Geometry check sheet. Reference: the model listing, model coordinates, mm. Give positions to 0.01 mm unless a question says otherwise; leave off trailing zeros. Write each loop counter-clockwise with the first axis right and the second up, starting at its lowest first coordinate (ties: lowest second). Pieces come first, ordered by that corner, then holes. Notation, with made-up numbers: M 32,8.5 L 65,8.5 A38 ccw 65,47.5 Z; hole C 46.25,75.5 d5. An arc over 180 degrees is marked long. One line per item, written item: value. Start each with the question number.
1. Scan lines: line 1 (Y direction, x = 32.5, z = 5); line 2 (X direction, y = -34, z = 3.75); line 3 (X direction, y = 53.5, z = 1). Record each from-to range of solid material in increasing order.
2. Gauge pin test, flat ends, axial feed: pin 1 (1.8 mm diameter, centred on x = -11, y = -54, fed in from -Z); pin 2 (2 mm diameter, centred on y = 58, z = 3.5, fed in from -X). Record the tip position at first contact, or that the pin passes through.
3. Cross-section at D-D on y = -29. Record the cut outline in (x, z).
4. Cross-section at A-A on y = 0. Record the cut outline in (x, z), then the cut area to 3 significant figures.
5. Cross-section at C-C on z = 4. Count the separate pieces of the cut face and the enclosed holes in it, then the cut area to 3 significant figures.
from build123d import *

# Parameters (mm, degrees)
SKETCH1_R           = 76.2
SKETCH1_R_2         = 2.25
SKETCH1_R_3         = 1.5
SKETCH1_R_4         = 1
SKETCH1_W           = 25.4
SKETCH1_H           = 25.4
BOSS_EXTRUDE2_DEPTH = 6.35
FILLET3_R           = 1
FILLET4_R           = 1
FILLET5_R           = 1
FILLET6_R           = 1


with BuildPart() as part:
    # Sketch1 → Boss-Extrude2 (new body)
    with BuildSketch(Plane.XY):
        Circle(SKETCH1_R)
        with Locations((-32.5, 29)):
            Circle(SKETCH1_R_2, mode=Mode.SUBTRACT)
        with Locations((-32.5, -29)):
            Circle(SKETCH1_R_2, mode=Mode.SUBTRACT)
        with Locations((32.5, -29)):
            Circle(SKETCH1_R_2, mode=Mode.SUBTRACT)
        with Locations((32.5, 29)):
            Circle(SKETCH1_R_2, mode=Mode.SUBTRACT)
        with Locations((43.5, 35)):
            Circle(SKETCH1_R_3, mode=Mode.SUBTRACT)
        with Locations((-43.5, 35)):
            Circle(SKETCH1_R_3, mode=Mode.SUBTRACT)
        with Locations((43.5, -35)):
            Circle(SKETCH1_R_3, mode=Mode.SUBTRACT)
        with Locations((-43.5, -35)):
            Circle(SKETCH1_R_3, mode=Mode.SUBTRACT)
        with Locations((-11, 54)):
            Circle(SKETCH1_R_4, mode=Mode.SUBTRACT)
        with Locations((11, 54)):
            Circle(SKETCH1_R_4, mode=Mode.SUBTRACT)
        with Locations((11, 62)):
            Circle(SKETCH1_R_4, mode=Mode.SUBTRACT)
        with Locations((-11, 62)):
            Circle(SKETCH1_R_4, mode=Mode.SUBTRACT)
        with Locations((-11, -62)):
            Circle(SKETCH1_R_4, mode=Mode.SUBTRACT)
        with Locations((-11, -54)):
            Circle(SKETCH1_R_4, mode=Mode.SUBTRACT)
        with Locations((11, -62)):
            Circle(SKETCH1_R_4, mode=Mode.SUBTRACT)
        with Locations((11, -54)):
            Circle(SKETCH1_R_4, mode=Mode.SUBTRACT)
        Rectangle(SKETCH1_W, SKETCH1_H, mode=Mode.SUBTRACT)
    extrude(amount=BOSS_EXTRUDE2_DEPTH)

    # Fillet3
    fillet3_edges = [part.edges().sort_by_distance(p)[0] for p in [
        (-12.7, -12.7, 3.175),
    ]]
    fillet(fillet3_edges, radius=FILLET3_R)

    # Fillet4
    fillet4_edges = [part.edges().sort_by_distance(p)[0] for p in [
        (12.7, 12.7, 3.175),
    ]]
    fillet(fillet4_edges, radius=FILLET4_R)

    # Fillet5
    fillet5_edges = [part.edges().sort_by_distance(p)[0] for p in [
        (-12.7, 12.7, 3.175),
    ]]
    fillet(fillet5_edges, radius=FILLET5_R)

    # Fillet6
    fillet6_edges = [part.edges().sort_by_distance(p)[0] for p in [
        (12.7, -12.7, 3.175),
    ]]
    fillet(fillet6_edges, radius=FILLET6_R)


solid = part.part
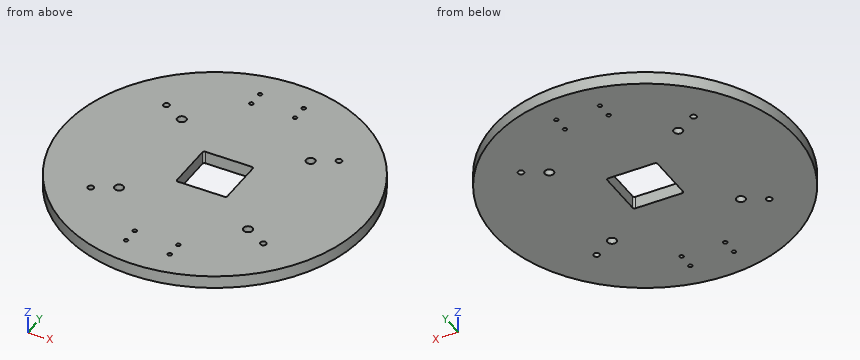
Report:
1. line 1: y = -68.92 to -31.25, -26.75 to 26.75, 31.25 to 68.92
1. line 2: x = -68.19 to -44.62, -42.38 to 42.38, 44.62 to 68.19
1. line 3: x = -54.26 to -11.87, -10.13 to 10.13, 11.87 to 54.26
2. pin 1: passes through
2. pin 2: stops at x = -50.57
3. outline: M -70.47,0 L -34.75,0 L -34.75,6.35 L -70.47,6.35 Z; M -30.25,0 L 30.25,0 L 30.25,6.35 L -30.25,6.35 Z; M 34.75,0 L 70.47,0 L 70.47,6.35 L 34.75,6.35 Z
4. outline: M -76.2,0 L -12.7,0 L -12.7,6.35 L -76.2,6.35 Z; M 12.7,0 L 76.2,0 L 76.2,6.35 L 12.7,6.35 Z
4. area: 806 mm^2
5. separate pieces: 1
5. enclosed holes: 17
5. area: 17,500 mm^2
